from build123d import *

# Parameters (mm, degrees)
BOSS_EXTRUDE1_DEPTH                                 = 178
CBORE_FOR_4_BINDING_HEAD_MACHINE_SCREW3_D           = 3.2639
CBORE_FOR_4_BINDING_HEAD_MACHINE_SCREW3_CBORE_D     = 6.74624
CBORE_FOR_4_BINDING_HEAD_MACHINE_SCREW3_CBORE_DEPTH = 1.7272
SKETCH3_R                                           = 1.397
CUT_EXTRUDE1_DEPTH                                  = 7.35
FILLET1_R                                           = 1.27


with BuildPart() as part:
    # Sketch2 → Boss-Extrude1 (new body)
    with BuildSketch(Plane(origin=(0, 0, 0), x_dir=(1, 0, 0), z_dir=(0, 1, 0))):
        with BuildLine():
            Line((8.001, -203.2), (-8.001, -203.2))
            Line((-8.001, -203.2), (-5.969, -196.937688608))
            ThreePointArc((-5.969, -196.937688608), (0, -196.85), (5.969, -196.937688608))
            Line((5.969, -196.937688608), (8.001, -203.2))
        make_face()
    extrude(amount=BOSS_EXTRUDE1_DEPTH)

    # CBORE for #4 Binding Head Machine Screw3 (through all)
    with Locations(Plane(origin=(0, 8, 196.85), x_dir=(-1, 0, 0), z_dir=(0, 0, -1))):
        with Locations((0, 0), (0, 137.875371205)):
            CounterBoreHole(CBORE_FOR_4_BINDING_HEAD_MACHINE_SCREW3_D / 2, CBORE_FOR_4_BINDING_HEAD_MACHINE_SCREW3_CBORE_D / 2, CBORE_FOR_4_BINDING_HEAD_MACHINE_SCREW3_CBORE_DEPTH)

    # Sketch3 → Cut-Extrude1 (cut, through all)
    with BuildSketch(Plane.XY.offset(196.85)):
        with Locations((0, 27)):
            Circle(SKETCH3_R)
        with Locations((0, 127)):
            Circle(SKETCH3_R)
    extrude(amount=CUT_EXTRUDE1_DEPTH, mode=Mode.SUBTRACT)

    # Fillet1
    fillet1_edges = [part.edges().sort_by_distance(p)[0] for p in [
        (8.001, 89, 203.2),
        (-8.001, 89, 203.2),
    ]]
    fillet(fillet1_edges, radius=FILLET1_R)


solid = part.part
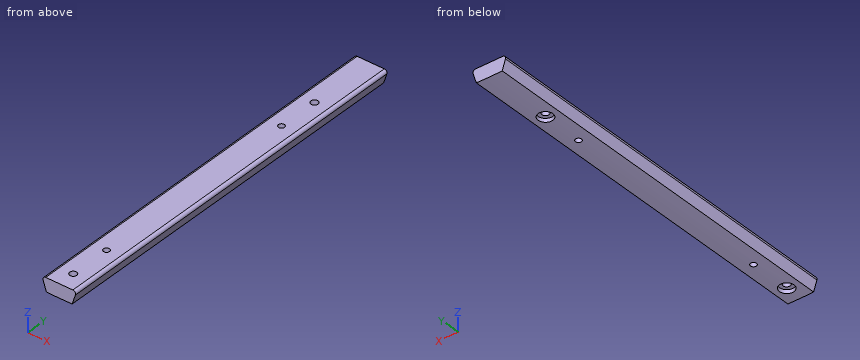
Check sheet for the modelled part. Datum: model origin and axes. Units: mm. Give positions to 0.01 mm unless a question says otherwise; leave off trailing zeros. Loops run counter-clockwise (first coordinate to the right, second up) from the corner with the lowest first, then second, coordinate; pieces in that order, holes last. Notation, with made-up numbers: M 62.25,62 L 99.25,62 A27 cw 99.25,90 Z; hole C -34.5,76 d1. An arc over 180 degrees is marked long. Return JSON: item names as keys, results as strings. Group by question number.
1. Go/stop test with flat-tipped pins: pin 1 (2.5 mm diameter, centred on x = 0, y = 127, fed in from -Z); pin 2 (3 mm diameter, centred on x = -4.5, y = 34.5, fed in from -Z); pin 3 (3.5 mm diameter, centred on x = -1, y = 145, fed in from -Z). Record where each tip stops, or that it passes through.
2. Cross-section at C-C on y = 151. Record the boundary of the cut face in (x, z), plus the area to 3 significant figures.
3. Cross-section at B-B on z = 200. Record the boundary of the cut face in (x, y), plus the area to 3 significant figures.
4. Cross-section at A-A on y = 8. Record the boundary of the cut face in (x, z).
5. Thickness scan on L1, parallel to Y at x = 0, z = 197.95; L2, parallel to Y at x = 0, z = 200.6; L3, parallel to Z at x = 3.5, y = 142.5. Record the ranges inside material, lowest first.
Return value:
{
 "1": {"pin 1": "through", "pin 2": "z = 196.87", "pin 3": "z = 198.58"},
 "2": {"outline": "M -7.46,201.54 L -5.97,196.94 A203.2 ccw 5.97,196.94 L 7.46,201.54 A1.27 ccw 6.25,203.2 L -6.25,203.2 A1.27 ccw Z", "area": "86.8 mm^2"},
 "3": {"outline": "M -6.96,0 L 6.96,0 L 6.96,178 L -6.96,178 Z; hole C 0,8 d3.26; hole C 0,145.88 d3.26; hole C 0,27 d2.79; hole C 0,127 d2.79", "area": "2,450 mm^2"},
 "4": {"outline": "M -7.46,201.54 L -5.97,196.94 A203.2 ccw -3.37,196.88 L -3.37,198.58 L -1.63,198.58 L -1.63,203.2 L -6.25,203.2 A1.27 ccw Z; M 1.63,198.58 L 3.37,198.58 L 3.37,196.88 A203.2 ccw 5.97,196.94 L 7.46,201.54 A1.27 ccw 6.25,203.2 L 1.63,203.2 Z"},
 "5": {"L1": "0 to 4.63, 11.37 to 25.6, 28.4 to 125.6, 128.4 to 142.5, 149.25 to 178", "L2": "0 to 6.37, 9.63 to 25.6, 28.4 to 125.6, 128.4 to 144.24, 147.51 to 178", "L3": "196.88 to 203.2"}
}
